Source: CAD feature listing. Evaluate the final solid. Frame: model axes, mm. A direction names the side the tool comes from. Round coordinates to 2 decimals unless told otherwise and drop trailing zeros. Order: outer loops, then holes, each group sorted by start corner. A loop starts at its lowest first (then second) coordinate and runs counter-clockwise, first axis right, second up. Notation, with made-up numbers: (47, 44) -> (82, 44) arc R7 cw to (82, 56) -> close; hole circle Ø5 at (43, 70.5). An arc over 180 degrees is marked (long way). Use a Markdown table: item, result. Add a question column.
```python
from build123d import *

# Parameters (mm, degrees)
F0_R      = 2.5
F0_W      = 20
F0_H      = 26
F0_H_2    = 7
F1_DEPTH  = 6
F0_W_2    = 95
F0_H_3    = 6
F2_DEPTH  = 25
F3_R      = 2.5
F4_DEPTH  = 25
F5_SIZE   = 5
F6_R      = 5
F7_DEPTH  = 25
F9_DEPTH  = 25
F10_R     = 1.75
F11_DEPTH = 50
F10_R_2   = 2.5
F12_DEPTH = 10
F13_R     = 2
F14_R     = 5
F15_R     = 5


with BuildPart() as f1:
    # F0 (on Top) → F1 (new body)
    with BuildSketch(Plane.XY):
        Polygon((-47.5, 20), (-47.5, 0), (-10, 0), (10, 0), (47.5, 0), (47.5, 20), align=None)
        with Locations((-37.5, 6.5)):
            Circle(F0_R, mode=Mode.SUBTRACT)
        with Locations((37.5, 6.5)):
            Circle(F0_R, mode=Mode.SUBTRACT)
        with Locations((0, -20)):
            Rectangle(F0_W, F0_H)
        with Locations((0, -36.5)):
            Rectangle(F0_W, F0_H_2)
        with Locations((0, -3.5)):
            Rectangle(F0_W, F0_H_2)
    extrude(amount=F1_DEPTH)

    # F0 (on Top) → F2 (join)
    with BuildSketch(Plane.XY):
        with Locations((0, 23)):
            Rectangle(F0_W_2, F0_H_3)
    extrude(amount=F2_DEPTH)

    # F3 (on face) → F4 (cut)
    with BuildSketch(Plane.XZ.offset(-20)):
        with Locations((-37.5, 17.5)):
            Circle(F3_R)
        with Locations((37.5, 17.5)):
            Circle(F3_R)
    extrude(amount=-F4_DEPTH, mode=Mode.SUBTRACT)

    # F5
    f5_edges = [f1.edges().sort_by_distance(p)[0] for p in [
        (0, 20, 6),
        (0, 26, 0),
    ]]
    chamfer(f5_edges, length=F5_SIZE)

    # F6
    f6_edges = [f1.edges().sort_by_distance(p)[0] for p in [
        (47.5, 23, 25),
        (47.5, 0, 3),
        (-47.5, 0, 3),
        (-47.5, 23, 25),
    ]]
    fillet(f6_edges, radius=F6_R)

    # F0 (on Top) → F7 (join)
    with BuildSketch(Plane.XY):
        with Locations((0, -3.5)):
            Rectangle(F0_W, F0_H_2)
        with Locations((0, -36.5)):
            Rectangle(F0_W, F0_H_2)
    extrude(amount=F7_DEPTH)

    # F8 (on face) → F9 (cut)
    with BuildSketch(Plane.YZ.offset(10)):
        with BuildLine():
            Line((-33, 10), (-33, 12))
            ThreePointArc((-33, 12), (-34, 11), (-33, 10))
        make_face()
        with BuildLine():
            Line((-7, 12), (-7, 10))
            ThreePointArc((-7, 10), (-6.2928932188, 10.2928932188), (-6, 11))
            ThreePointArc((-6, 11), (-6.2928932188, 11.7071067812), (-7, 12))
        make_face()
    extrude(amount=-F9_DEPTH, mode=Mode.SUBTRACT)

    # F10 (on face) → F11 (cut)
    with BuildSketch(Plane.XZ.offset(7)):
        with Locations((0, 20)):
            Circle(F10_R)
    extrude(amount=F11_DEPTH, mode=Mode.SUBTRACT)

    # F10 (on face) → F12 (cut)
    with BuildSketch(Plane.XZ.offset(7)):
        with Locations((0, 20)):
            Circle(F10_R_2)
        with Locations((0, 20)):
            Circle(F10_R, mode=Mode.SUBTRACT)
        with Locations((0, 20)):
            Circle(F10_R)
    extrude(amount=-F12_DEPTH, mode=Mode.SUBTRACT)

    # F13
    f13_edges = [f1.edges().sort_by_distance(p)[0] for p in [
        (0, -7, 25),
        (0, 0, 25),
        (0, -33, 25),
        (0, -40, 25),
        (0, -40, 0),
    ]]
    fillet(f13_edges, radius=F13_R)

    # F14
    f14_edges = [f1.edges().sort_by_distance(p)[0] for p in [
        (0, 0, 6),
    ]]
    fillet(f14_edges, radius=F14_R)

    # F15
    f15_edges = [f1.edges().sort_by_distance(p)[0] for p in [
        (10, 0, 3),
        (-10, 0, 3),
    ]]
    fillet(f15_edges, radius=F15_R)


solid = f1.part
```
1) Reachability of faces 4 (the cylindrical face through (-0.228, -36.451, 21.735)), 5 (the flat face through (29, 0, 3)), 6 (the flat face through (0, -33, 17)) from +Z, -Z, +X, -X, +Y, -Y: full face, straight path, thin tool, end or side. Return the list, or none.
2) Section A-A on x = -37.5. Output: boundary loops of the cut face in (y, z).
3) Draft query along X for faces 1 (the cylindrical face through (-46.07, 1.5, 3.04)), 2 (the cylindrical face through (-35.115, 22.958, 18.251)), 3 (the flat face through (1, 17, 8)). Return one class per face: pulls with the +X half, pulls with the -X half, needs draft (parallel to the pull), parting line crosses it, or undercut.
4) First-contact query: pin 1 Ø5 at (x, y) = (-24.5, 8.5) entering from +Z; pin 2 Ø1.8 at (x, z) = (22, 2.5) entering from -Y; pin 3 Ø1 at (y, z) = (-10, 7) entering from -X; pin 4 Ø6.5 at (x, z) = (37.5, 17.5) entering from -Y. Flat tips, straight axial feed; report the tip coordinate or a pass-through.
5) Line query: probe 1 along Z at (x, y) = (0, -38); probe 2 along X at (y, z) = (7, 5); probe 3 along Y at (x, z) = (-37.5, 2). Output: solid intervals per line, ascending. Write a range as from..to.
6) Section B-B on x = 21. Output: boundary loops of the cut face in (y, z), then the cut area to 3 significant figures.
7) Section C-C on x = 0. Count the separate pieces of the cut face and the enclosed holes in it, then the cut area to 3 significant figures.
8) Section D-D on y = 14. Output: boundary loops of the cut face in (x, z).
Conclusion:
| question | item | result |
|---|---|---|
| 1 | face 4 | -Y |
| 1 | face 5 | +Z, -Z, +X, -Y |
| 1 | face 6 | +Z, +X, -X |
| 2 | outline | (0, 0) -> (4, 0) -> (4, 6) -> (0, 6) -> close; (9, 0) -> (21, 0) -> (26, 5) -> (26, 15) -> (20, 15) -> (20, 11) -> (15, 6) -> (9, 6) -> close; (20, 20) -> (26, 20) -> (26, 25) -> (20, 25) -> close |
| 3 | face 1 | pulls with the -X half |
| 3 | face 2 | undercut |
| 3 | face 3 | needs draft |
| 4 | pin 1 | stops at z = 6 |
| 4 | pin 2 | stops at y = 0 |
| 4 | pin 3 | passes through |
| 4 | pin 4 | stops at y = 20 |
| 5 | probe 1 | z = 0..18.25, 21.75..25 |
| 5 | probe 2 | x = -47.5..-39.95, -35.05..35.05, 39.95..47.5 |
| 5 | probe 3 | y = 0..4, 9..23 |
| 6 | outline | (0, 0) -> (21, 0) -> (26, 5) -> (26, 25) -> (20, 25) -> (20, 11) -> (15, 6) -> (0, 6) -> close |
| 6 | area | 270 mm^2 |
| 7 | separate pieces | 3 |
| 7 | enclosed holes | 0 |
| 7 | area | 714 mm^2 |
| 8 | outline | (-47.5, 0) -> (47.5, 0) -> (47.5, 6) -> (-47.5, 6) -> close |
